Check sheet for the drawn part. Datum: minimum x, y, z corner. Units: mm. Round coordinates to 2 decimals unless told otherwise and drop trailing zeros. Write each loop counter-clockwise with the first axis right and the second up, starting at its lowest first coordinate (ties: lowest second). Pieces come first, ordered by that corner, then holes.
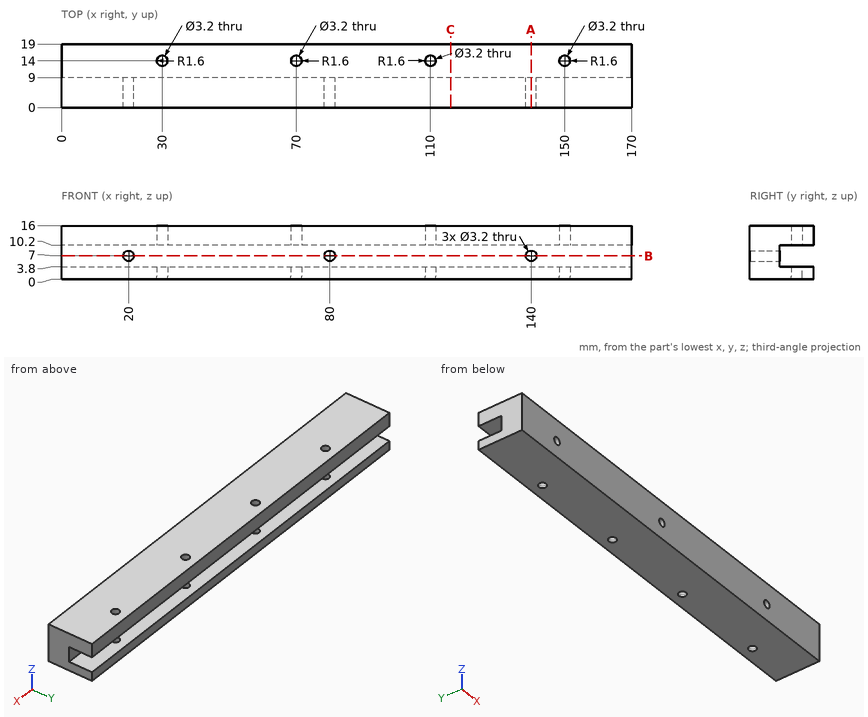
1. Go/stop test with flat-tipped pins: pin 1 (4 mm diameter, centred on x = 107.5, y = 5, fed in from -Z); pin 2 (1.9 mm diameter, centred on x = 80, z = 7, fed in from +Y). Record where each tip stops, or that it passes through.
2. Sectioned sample at A-A, the plane x = 140. Enter the section's corners in (y, z).
3. Sectioned sample at B-B, the plane z = 7. Enter the section's corners in (x, y).
4. Scan lines: line 1 along X through (y, z) = (14, 11.65); line 2 along X through (y, z) = (2.4, 7); line 3 along Z through (x, y) = (112.5, 14.5). Record each from-to range of solid material in increasing order.
5. Sectioned sample at C-C, the plane x = 116. Enter the section's corners in (y, z).
Computed values:
1. pin 1: stops at z = 0
1. pin 2: passes through
2. outline: (0, 0) - (19, 0) - (19, 3.8) - (9, 3.8) - (9, 5.4) - (0, 5.4) - close; (0, 8.6) - (9, 8.6) - (9, 10.2) - (19, 10.2) - (19, 16) - (0, 16) - close
3. outline: (0, 0) - (18.4, 0) - (18.4, 9) - (0, 9) - close; (21.6, 0) - (78.4, 0) - (78.4, 9) - (21.6, 9) - close; (81.6, 0) - (138.4, 0) - (138.4, 9) - (81.6, 9) - close; (141.6, 0) - (170, 0) - (170, 9) - (141.6, 9) - close
4. line 1: x = 0 to 28.4, 31.6 to 68.4, 71.6 to 108.4, 111.6 to 148.4, 151.6 to 170
4. line 2: x = 0 to 18.4, 21.6 to 78.4, 81.6 to 138.4, 141.6 to 170
4. line 3: z = 0 to 3.8, 10.2 to 16
5. outline: (0, 0) - (19, 0) - (19, 3.8) - (9, 3.8) - (9, 10.2) - (19, 10.2) - (19, 16) - (0, 16) - close
